```python
from build123d import *

# Parameters (mm, degrees)
SKETCH1_W           = 12.7
SKETCH1_H           = 12.7
SKETCH1_R           = 1.25
BOSS_EXTRUDE1_DEPTH = 3.175
SKETCH2_W           = 6.35
SKETCH2_H           = 1
BOSS_EXTRUDE2_DEPTH = 1.75


with BuildPart() as part:
    # Sketch1 → Boss-Extrude1 (new body, symmetric)
    with BuildSketch(Plane(origin=(0, 0, 0), x_dir=(1, 0, 0), z_dir=(0, 1, 0))):
        Rectangle(SKETCH1_W, SKETCH1_H)
        with Locations((-3.81, 0)):
            Circle(SKETCH1_R, mode=Mode.SUBTRACT)
        with Locations((3.81, 0)):
            Circle(SKETCH1_R, mode=Mode.SUBTRACT)
    extrude(amount=BOSS_EXTRUDE1_DEPTH, both=True)

    # Sketch2 → Boss-Extrude2 (add, symmetric)
    with BuildSketch(Plane(origin=(0, 0, 0), x_dir=(1, 0, 0), z_dir=(0, 1, 0))):
        with Locations((9.525, 3)):
            Rectangle(SKETCH2_W, SKETCH2_H)
        with Locations((9.525, -3)):
            Rectangle(SKETCH2_W, SKETCH2_H)
    extrude(amount=BOSS_EXTRUDE2_DEPTH, both=True)


solid = part.part
```
Input: part model. Units: mm. Frame: model coordinates. A direction names the side the tool comes from. Give positions to 0.01 mm unless a question says otherwise; leave off trailing zeros. Loops run counter-clockwise (first coordinate to the right, second up) from the corner with the lowest first, then second, coordinate; pieces in that order, holes last.
1) Mould query, pull axis Z, two halves, no side actions, for faces 4 (the flat face through (9, 0, 2.5)), 5 (the flat face through (9, -1.75, 3)), 6 (the flat face through (0, 0, -6.35)), 7 (the cylindrical face through (-5.06, -0.04, -0.05)). Classes: released by +Z, released by -Z, zero draft, split by the parting line, or undercut.
A:
face 4: undercut
face 5: zero draft
face 6: released by -Z
face 7: undercut
2) Section query A-A on z = 0. Return the cut outline in (x, y) (3 decimals), and give its area (3 significant figures).
A:
outline: (-6.35, -3.175) - (-5.06, -3.175) - (-5.06, 3.175) - (-6.35, 3.175) - close; (-2.56, -3.175) - (2.56, -3.175) - (2.56, 3.175) - (-2.56, 3.175) - close; (5.06, -3.175) - (6.35, -3.175) - (6.35, 3.175) - (5.06, 3.175) - close
area: 48.9 mm2
3) Section query B-B on x = 7. Return the cut outline in (y, z).
A:
outline: (-1.75, -3.5) - (1.75, -3.5) - (1.75, -2.5) - (-1.75, -2.5) - close; (-1.75, 2.5) - (1.75, 2.5) - (1.75, 3.5) - (-1.75, 3.5) - close
4) Contact query for flat-ended pins moving along their axis: pin 1 (0.8 mm diameter, centred on x = 11, z = -3, fed in from +Y); pin 2 (1 mm diameter, centred on x = 10, y = 0, fed in from +Z); pin 3 (1.8 mm diameter, centred on x = 10.5, y = 0.5, fed in from -Z). Output: stop coordinate, or through.
A:
pin 1: stops at y = 1.75
pin 2: stops at z = 3.5
pin 3: stops at z = -3.5
5) Section query C-C on y = 1.5. Return the cut outline in (x, z), and give its area (3 significant figures).
A:
outline: (-6.35, -6.35) - (6.35, -6.35) - (6.35, -3.5) - (12.7, -3.5) - (12.7, -2.5) - (6.35, -2.5) - (6.35, 2.5) - (12.7, 2.5) - (12.7, 3.5) - (6.35, 3.5) - (6.35, 6.35) - (-6.35, 6.35) - close; hole circle Ø2.5 at (-3.81, 0); hole circle Ø2.5 at (3.81, 0)
area: 164 mm2
6) Line query: L1, parallel to X at y = 0.75, z = 0; L2, parallel to Z at x = -3.81, y = -1.25; L3, parallel to Z at x = 6.5, y = 1. Output: solid intervals per line, ascending.
A:
L1: x = -6.35 to -5.06, -2.56 to 2.56, 5.06 to 6.35
L2: z = -6.35 to -1.25, 1.25 to 6.35
L3: z = -3.5 to -2.5, 2.5 to 3.5
7) Reachability of faces 1 (the flat face through (9, 0, 3.5)), 2 (the flat face through (9, -1.75, -3)), 3 (the flat face through (9, 0, -2.5)) from +Z, -Z, +X, -X, +Y, -Y: full face, straight path, thin tool, end or side. Return the list, or none.
A:
face 1: +Z, +X, +Y, -Y
face 2: +Z, -Z, +X, -Y
face 3: +X, +Y, -Y
8) Section query D-D on z = 3. Return the cut outline in (x, y) (3 decimals).
A:
outline: (-6.35, -3.175) - (6.35, -3.175) - (6.35, -1.75) - (12.7, -1.75) - (12.7, 1.75) - (6.35, 1.75) - (6.35, 3.175) - (-6.35, 3.175) - close
